For this review, use the dimensioned drawing (mm, ordinates from the lowest corner) and the shaded views. A direction names the side the tool comes from. Round coordinates to 2 decimals unless told otherwise and drop trailing zeros. Loops run counter-clockwise (first coordinate to the right, second up) from the corner with the lowest first, then second, coordinate; pieces in that order, holes last. Notation, with made-up numbers: M 54,36.5 L 63,36.5 A21 cw 63,41.5 Z; hole C 34.25,-20.5 d2. An arc over 180 degrees is marked long. Use a Markdown table: item, result. Add a question column.
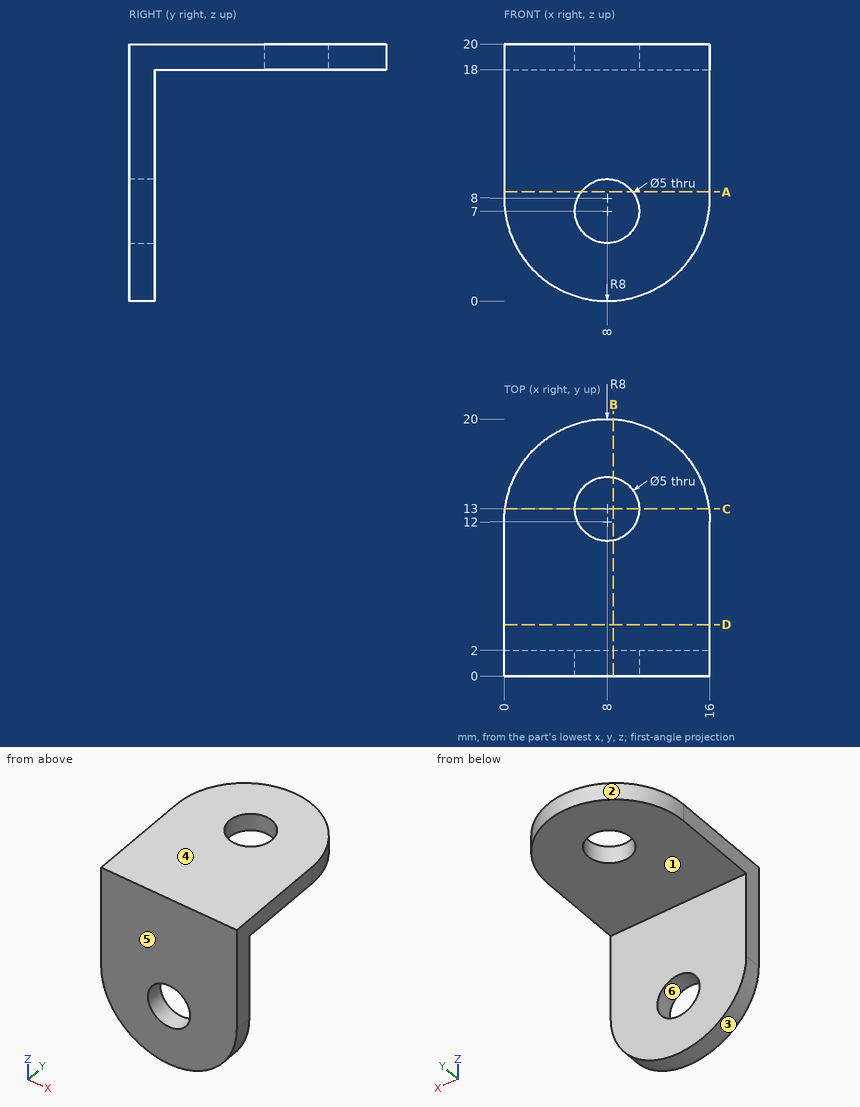
(1) Consider section D-D, the plane y = 4. Give the boundary of the cut face in (x, z), then the cut area to 3 significant figures.
(2) Consider section A-A, the plane z = 8.5. Give the boundary of the cut face in (x, y), then the cut area to 3 significant figures.
(3) To check wall thickness, follow probe 1 along Z at (x, y) = (8, 0.85); probe 2 along Y at (x, z) = (11.75, 16); probe 3 along Z at (x, y) = (7.75, 6.25). State the ranges of each line that lie inside material, in increasing order.
(4) Consider section C-C, the plane y = 13. Give the boundary of the cut face in (x, z), then the cut area to 3 significant figures.
(5) Draft analysis for pull direction Z (two halves, no side actions). For the marked faces 3, 4, 5 and 6, state which applies: released by +Z, released by -Z, zero draft, split by the parting line, or undercut.
(6) Consider section B-B, the plane x = 8.5. Give the boundary of the cut face in (y, z), then the cut area to 3 significant figures.
(7) For the marked faces 1 and 2, list the 3-axis set-ups (+Z, -Z, +X, -X, +Y, -Y) from which the entire face can be reached by the end or side of a thin tool; tool diameter is ignored.
(8) Insertion check: pin 1 Ø3 at (x, y) = (3, 11.5) entering from -Z; pin 2 Ø6 at (x, y) = (13, 3) entering from -Z. Each pin has a flat end and moves straight along its axis. Give the tip position at first contact, or say it passes through.
Found:
| question | item | result |
|---|---|---|
| 1 | outline | M 0,18 L 16,18 L 16,20 L 0,20 Z |
| 1 | area | 32.0 mm^2 |
| 2 | outline | M 0,0 L 6,0 L 6,2 L 0,2 Z; M 10,0 L 16,0 L 16,2 L 10,2 Z |
| 2 | area | 24.0 mm^2 |
| 3 | probe 1 | z = 0 to 4.5, 9.5 to 20 |
| 3 | probe 2 | y = 0 to 2 |
| 3 | probe 3 | z = 18 to 20 |
| 4 | outline | M 0.06,18 L 5.5,18 L 5.5,20 L 0.06,20 Z; M 10.5,18 L 15.94,18 L 15.94,20 L 10.5,20 Z |
| 4 | area | 21.7 mm^2 |
| 5 | face 3 | released by -Z |
| 5 | face 4 | released by +Z |
| 5 | face 5 | zero draft |
| 5 | face 6 | undercut |
| 6 | outline | M 0,0.02 L 2,0.02 L 2,4.55 L 0,4.55 Z; M 0,9.45 L 2,9.45 L 2,18 L 10.55,18 L 10.55,20 L 0,20 Z; M 15.45,18 L 19.98,18 L 19.98,20 L 15.45,20 Z |
| 6 | area | 56.3 mm^2 |
| 7 | face 1 | -Z, +X, -X, +Y |
| 7 | face 2 | +Z, -Z, +Y |
| 8 | pin 1 | stops at z = 18 |
| 8 | pin 2 | stops at z = 0.3 |
